from build123d import *

# Parameters (mm, degrees)
SKETCH1_W             = 15.24
SKETCH1_H             = 12.7
MAIN_BASE_DEPTH       = 2.54
ALIGNMENTPINS_START   = 1.778
SKETCH2_R             = 0.381
ALIGNMENTPINS_DEPTH   = 1.27
ALIGNMENTPINS_2_DEPTH = 1.27
SKETCH7_W             = 7.62
SKETCH7_H             = 12.7
PCBOARDEDGES_DEPTH    = 1.778
SKETCH12_W            = 4.379010271
SKETCH12_H            = 3.048
CONNECTORALIGN_DEPTH  = 2.54
SKETCH13_W            = 3.302
SKETCH13_H            = 5.08
LEDHOLE_DEPTH         = 5.318
SKETCH14_W            = 11.999010271
SKETCH14_H            = 6.858
SHOULDER_DEPTH        = 2.54
SKETCH15_W            = 11.999010271
SKETCH15_H            = 6.858
SHOULDER2_DEPTH       = 2.54
PCB_CLIP_START        = -4.37901
SKETCH17_R            = 0.254
PCB_CLIP_DEPTH        = 4.37901
SKETCH18_W            = 4.572
SKETCH18_H            = 2.54
NUNCHUCKCLIP_DEPTH    = 1.27
SKETCH19_W            = 4.572
SKETCH19_H            = 2.54
NUNCHUCKCLIP2_DEPTH   = 1.27
CUT_EXTRUDE1_DEPTH    = 0.508


with BuildPart() as part:
    # Sketch1 → Main Base (new body)
    with BuildSketch(Plane(origin=(0, 0, 0), x_dir=(1, 0, 0), z_dir=(0, 1, 0))):
        with Locations((7.62, 6.35)):
            Rectangle(SKETCH1_W, SKETCH1_H)
    extrude(amount=MAIN_BASE_DEPTH)



with BuildPart() as body_2:
    # Sketch2 → AlignmentPins (new body)
    with BuildSketch(Plane(origin=(0, 2.54, 0), x_dir=(-1, 0, 0), z_dir=(0, 1, 0)).offset(ALIGNMENTPINS_START)):
        with Locations((-0.762, -6.35)):
            Circle(SKETCH2_R)
    extrude(amount=ALIGNMENTPINS_DEPTH)


with BuildPart() as body_3:
    # Sketch2 → AlignmentPins 2 (new body)
    with BuildSketch(Plane(origin=(0, 2.54, 0), x_dir=(-1, 0, 0), z_dir=(0, 1, 0)).offset(ALIGNMENTPINS_START)):
        with Locations((-5.588, -6.35)):
            Circle(SKETCH2_R)
    extrude(amount=ALIGNMENTPINS_2_DEPTH)


with BuildPart() as part_1:
    add(part.part)

    add(body_2.part)  # PCBoardEdges merges body 2

    add(body_3.part)  # PCBoardEdges merges body 3
    # Sketch7 → PCBoardEdges (add)
    with BuildSketch(Plane(origin=(0, 2.54, 0), x_dir=(1, 0, 0), z_dir=(0, 1, 0))):
        with Locations((3.81, 6.35)):
            Rectangle(SKETCH7_W, SKETCH7_H)
    extrude(amount=PCBOARDEDGES_DEPTH)

    # Sketch12 → ConnectorAlign (add)
    with BuildSketch(Plane(origin=(0, 4.318, 0), x_dir=(1, 0, 0), z_dir=(0, 1, 0))):
        with Locations((5.430494864, 1.524)):
            Rectangle(SKETCH12_W, SKETCH12_H)
        with Locations((5.430494864, 11.176)):
            Rectangle(SKETCH12_W, SKETCH12_H)
    extrude(amount=CONNECTORALIGN_DEPTH)

    # Sketch13 → LEDHole (cut, through all)
    with BuildSketch(Plane(origin=(0, 4.318, 0), x_dir=(1, 0, 0), z_dir=(0, 1, 0))):
        with Locations((3.175, 6.35)):
            Rectangle(SKETCH13_W, SKETCH13_H)
    extrude(amount=-LEDHOLE_DEPTH, mode=Mode.SUBTRACT)

    # Sketch14 → Shoulder (add)
    with BuildSketch(Plane.XY):
        with Locations((9.240494865, 3.429)):
            Rectangle(SKETCH14_W, SKETCH14_H)
    extrude(amount=SHOULDER_DEPTH)

    # Sketch15 → Shoulder2 (add)
    with BuildSketch(Plane(origin=(0, 0, -12.7), x_dir=(-1, 0, 0), z_dir=(0, 0, -1))):
        with Locations((-9.240494865, 3.429)):
            Rectangle(SKETCH15_W, SKETCH15_H)
    extrude(amount=SHOULDER2_DEPTH)

    # Sketch17 → PCB_Clip (add)
    with BuildSketch(Plane(origin=(7.62, 0, 0), x_dir=(0, 0, -1), z_dir=(1, 0, 0)).offset(PCB_CLIP_START)):
        with Locations((3.048, 6.477)):
            Circle(SKETCH17_R)
        with Locations((9.652, 6.477)):
            Circle(SKETCH17_R)
    extrude(amount=PCB_CLIP_DEPTH)

    # Sketch18 → NunchuckClip (cut)
    with BuildSketch(Plane(origin=(0, 0, 0), x_dir=(-1, 0, 0), z_dir=(0, 0, -1))):
        with Locations((-9.906, 5.588)):
            Rectangle(SKETCH18_W, SKETCH18_H)
    extrude(amount=-NUNCHUCKCLIP_DEPTH, mode=Mode.SUBTRACT)

    # Sketch19 → NunchuckClip2 (cut)
    with BuildSketch(Plane.XY.offset(-12.7)):
        with Locations((9.906, 5.588)):
            Rectangle(SKETCH19_W, SKETCH19_H)
    extrude(amount=-NUNCHUCKCLIP2_DEPTH, mode=Mode.SUBTRACT)

    # Sketch20 → Cut-Extrude1 (cut)
    with BuildSketch(Plane.XZ):
        Polygon((8.217257779, -3.407193662), (8.217257779, -5.712243662), (6.016982779, -5.712243662), (6.016982779, -0.892593662), (14.398982779, -0.892593662), (14.398982779, -5.712243662), (12.198707779, -5.712243662), (12.198707779, -3.407193662), (11.255732779, -3.407193662), (11.255732779, -5.083593662), (9.055457779, -5.083593662), (9.055457779, -3.407193662), align=None)
        with BuildLine():
            Line((14.398982779, -7.493418662), (14.398982779, -11.893968662))
            Line((14.398982779, -11.893968662), (12.932132779, -11.893968662))
            Line((12.932132779, -11.893968662), (12.932132779, -9.819751084))
            Line((12.932132779, -9.819751084), (11.781244888, -9.62002374))
            add(Edge.make_bspline(
                [(11.781244888, -9.62002374), (11.770251243, -9.701615614), (11.748663963, -9.861830588), (11.690486481, -10.092391141), (11.615599165, -10.308891021), (11.520125231, -10.50985122), (11.405471862, -10.695560634), (11.270958242, -10.865311588), (11.120486873, -11.022229739), (10.949196623, -11.16103415), (10.761135353, -11.283987594), (10.557944594, -11.392930954), (10.337872373, -11.481879106), (10.102990479, -11.555971833), (9.853586477, -11.614857534), (9.588035638, -11.655012226), (9.307512918, -11.680069087), (9.114994844, -11.682943238), (9.016167154, -11.684418662)],
                knots=[0, 0, 0, 0, 0.000246818, 0.000484656, 0.000711955, 0.000933104, 0.001150717, 0.001365234, 0.001581735, 0.001801627, 0.002025024, 0.00225499, 0.002492123, 0.002735986, 0.002993304, 0.003260037, 0.003541058, 0.003837488, 0.003837488, 0.003837488, 0.003837488], degree=3))
            add(Edge.make_bspline(
                [(9.016167154, -11.684418662), (8.905845682, -11.682210565), (8.68961718, -11.677882727), (8.372872854, -11.644171577), (8.070289394, -11.591506566), (7.783499686, -11.513120981), (7.50963283, -11.418624818), (7.253853676, -11.294705499), (7.009895928, -11.155322531), (6.785472567, -10.99155228), (6.581476114, -10.81250602), (6.401376691, -10.621361865), (6.251345496, -10.416180814), (6.127577636, -10.200488598), (6.029896075, -9.973283881), (5.961530212, -9.734567465), (5.918899529, -9.48458455), (5.914467439, -9.314058562), (5.912207779, -9.22711749)],
                knots=[0, 0, 0, 0, 0.000330895, 0.000648549, 0.000954583, 0.00125123, 0.001539645, 0.00182231, 0.002102538, 0.002381539, 0.002654132, 0.002915916, 0.003167717, 0.003414839, 0.003660542, 0.00390768, 0.004158249, 0.004418878, 0.004418878, 0.004418878, 0.004418878], degree=3))
            add(Edge.make_bspline(
                [(5.912207779, -9.22711749), (5.91445515, -9.141879038), (5.918894654, -8.973497236), (5.952975516, -8.724244798), (6.006861153, -8.48157511), (6.081680985, -8.244815631), (6.181740166, -8.016042881), (6.300749021, -7.793180228), (6.443204901, -7.577175879), (6.60469356, -7.3712837), (6.778629295, -7.179505186), (6.962203599, -7.01236275), (7.15024709, -6.869703261), (7.343165184, -6.752025997), (7.544148349, -6.663616031), (7.748263448, -6.596817328), (7.959336029, -6.558322833), (8.101419593, -6.553084662), (8.173055826, -6.550443662)],
                knots=[0, 0, 0, 0, 0.000255646, 0.000505008, 0.000753251, 0.00100073, 0.001248584, 0.001501277, 0.001757823, 0.002023741, 0.002285618, 0.002533617, 0.002767397, 0.002992849, 0.00320977, 0.003424631, 0.003635926, 0.003850787, 0.003850787, 0.003850787, 0.003850787], degree=3))
            add(Edge.make_bspline(
                [(8.173055826, -6.550443662), (8.185703613, -6.55112084), (8.209065854, -6.552371684), (8.21468206, -6.574619572), (8.217257779, -6.584822959)],
                knots=[0, 0, 0, 0, 3.375e-05, 6.2341e-05, 6.2341e-05, 6.2341e-05, 6.2341e-05], degree=3))
            add(Edge.make_bspline(
                [(8.217257779, -6.584822959), (8.21379986, -6.598956726), (8.204910316, -6.635291506), (8.178023964, -6.661887625), (8.16159606, -6.678138193)],
                knots=[0, 0, 0, 0, 4.2972e-05, 0.000110472, 0.000110472, 0.000110472, 0.000110472], degree=3))
            add(Edge.make_bspline(
                [(8.16159606, -6.678138193), (8.136365772, -6.700405265), (8.077016572, -6.752784095), (7.993692338, -6.862131275), (7.902122779, -7.009388757), (7.800385555, -7.184339204), (7.708056874, -7.377085557), (7.639849213, -7.574659381), (7.596386201, -7.767637982), (7.591153517, -7.895938561), (7.588607779, -7.958357724)],
                knots=[0, 0, 0, 0, 0.000100772, 0.000237046, 0.000410069, 0.00062125, 0.000843879, 0.001049934, 0.0012474, 0.00143449, 0.00143449, 0.00143449, 0.00143449], degree=3))
            add(Edge.make_bspline(
                [(7.588607779, -7.958357724), (7.589364169, -8.003161205), (7.590845457, -8.090902724), (7.607861397, -8.218508769), (7.633961608, -8.339043342), (7.670022293, -8.453352628), (7.717335918, -8.560860294), (7.774738157, -8.661469601), (7.843243248, -8.754458019), (7.920801372, -8.840377114), (8.008056037, -8.917894183), (8.103416935, -8.984707761), (8.204925166, -9.042944891), (8.314460725, -9.087724989), (8.428623769, -9.127224479), (8.551689353, -9.149790175), (8.680576304, -9.167789672), (8.76943719, -9.169132909), (8.814802701, -9.169818662)],
                knots=[0, 0, 0, 0, 0.000134333, 0.000263072, 0.000385418, 0.000503982, 0.000622001, 0.000737136, 0.000850758, 0.00096782, 0.00108379, 0.001200071, 0.001316628, 0.001433998, 0.001554623, 0.001678233, 0.001808597, 0.001944566, 0.001944566, 0.001944566, 0.001944566], degree=3))
            add(Edge.make_bspline(
                [(8.814802701, -9.169818662), (8.855799497, -9.169091152), (8.935958333, -9.16766869), (9.052576868, -9.150249952), (9.16328584, -9.125037681), (9.265814181, -9.086505827), (9.363252497, -9.041250504), (9.451262049, -8.981147756), (9.533643551, -8.912152178), (9.609276284, -8.833428845), (9.67666913, -8.744332428), (9.73502713, -8.646476727), (9.785210532, -8.540365748), (9.823615634, -8.425214765), (9.85492271, -8.301566212), (9.87766612, -8.169699968), (9.890636219, -8.029012368), (9.892629227, -7.932736654), (9.893657779, -7.883050693)],
                knots=[0, 0, 0, 0, 0.000122881, 0.000240263, 0.000353034, 0.00046283, 0.000568268, 0.000674516, 0.000781419, 0.000890259, 0.001001257, 0.001115807, 0.001231522, 0.001352668, 0.00147933, 0.001613902, 0.001753672, 0.001902729, 0.001902729, 0.001902729, 0.001902729], degree=3))
            add(Edge.make_bspline(
                [(9.893657779, -7.883050693), (9.892472166, -7.825689716), (9.890150122, -7.713347192), (9.869778513, -7.548529099), (9.837864771, -7.391618982), (9.791184949, -7.242714697), (9.733050352, -7.101808236), (9.65950445, -6.969728078), (9.575093218, -6.844330987), (9.508174474, -6.768579517), (9.474557779, -6.730525693)],
                knots=[0, 0, 0, 0, 0.000172021, 0.000336907, 0.000497444, 0.000651749, 0.000804378, 0.000953849, 0.001104606, 0.001256786, 0.001256786, 0.001256786, 0.001256786], degree=3))
            Line((9.474557779, -6.730525693), (9.536767935, -6.655218662))
            Line((9.536767935, -6.655218662), (14.398982779, -7.493418662))
        make_face()
    extrude(amount=-CUT_EXTRUDE1_DEPTH, mode=Mode.SUBTRACT)


solid = part_1.part
Input: part model. Units: mm. Frame: model coordinates. A direction names the side the tool comes from. Coordinates: 2 decimals unless noted, no trailing zeros. Loops run counter-clockwise (first coordinate to the right, second up) from the corner with the lowest first, then second, coordinate; pieces in that order, holes last. Notation, with made-up numbers: (7.25, 35) -> (54.25, 35) arc R14 ccw to (54.25, 41) -> close; hole circle Ø10 at (-21.5, 68). An arc over 180 degrees is marked (long way). Write item = value, one per line. Start each with the question number.
Item 1: First-contact query: P1, Ø6, axis at x = 10, z = -9, coming from the +Y side; P2, Ø4, axis at y = 5, z = -4, coming from the +X side; P3, Ø1.4, axis at y = 5.5, z = -13, coming from the -X side; P4, Ø4, axis at x = 11.5, z = -3, coming from the +Y side. Flat tips, straight axial feed; report the tip coordinate or a pass-through.
Item 2: Reachability of faces 4 (the face through (3, 2, -3.81)), 5 (the face through (12, 4, 0)), 6 (the face through (10, 4.318, 1)), 7 (the face through (10, 0.508, -9)) from +Z, -Z, +X, -X, +Y, -Y: full face, straight path, thin tool, end or side. Return the list, or none.
Item 3: Cut plane C-C, the plane z = 0.75. Return loops of the section in (x, y), plus the area to 3 significant figures.
Item 4: Cut plane A-A, the plane z = -4.5. Return loops of the section in (x, y), plus the area to 3 significant figures.
Item 5: Mould query, pull axis X, two halves, no side actions, for faces 1 (the face through (15.24, 2, -6)), 2 (the face through (5, 5, -3.048)), 3 (the face through (4.826, 2, -6)). Classes: pulls with the +X half, pulls with the -X half, needs draft (parallel to the pull), parting line crosses it, or undercut.
Item 6: Cut plane D-D, the plane z = -6.35. Return loops of the section in (x, y).
Item 7: Cut plane B-B, the plane y = 2.75. Return loops of the section in (x, z).
Item 8: Material intervals for line 1 (Z direction, x = 13.75, y = 3.25); line 2 (X direction, y = 2.5, z = -6); line 3 (Z direction, x = 3, y = 3), sorted ascending.
Ans:
q1.P1 = 6.86
q1.P2 = 7.62
q1.P3 = 3.24
q1.P4 = 2.54
q2.face_4 = +Y, -Y
q2.face_5 = +X, +Y
q2.face_6 = +Y
q2.face_7 = -Y
q3.outline = (3.24, 0) -> (15.24, 0) -> (15.24, 6.86) -> (12.19, 6.86) -> (12.19, 4.32) -> (7.62, 4.32) -> (7.62, 6.86) -> (3.24, 6.86) -> close
q3.area = 70.7 mm²
q4.outline = (0, 0) -> (1.52, 0) -> (1.52, 4.32) -> (0, 4.32) -> close; (4.83, 0) -> (6.02, 0) -> (6.02, 0.51) -> (8.22, 0.51) -> (8.22, 0) -> (9.06, 0) -> (9.06, 0.51) -> (11.26, 0.51) -> (11.26, 0) -> (12.2, 0) -> (12.2, 0.51) -> (14.4, 0.51) -> (14.4, 0) -> (15.24, 0) -> (15.24, 2.54) -> (7.62, 2.54) -> (7.62, 4.32) -> (4.83, 4.32) -> close
q4.area = 34.6 mm²
q5.face_1 = pulls with the +X half
q5.face_2 = needs draft
q5.face_3 = undercut
q6.outline = (0, 0) -> (1.52, 0) -> (1.52, 4.32) -> (1.14, 4.32) -> (1.14, 5.59) -> (0.38, 5.59) -> (0.38, 4.32) -> (0, 4.32) -> close; (4.83, 0) -> (15.24, 0) -> (15.24, 2.54) -> (7.62, 2.54) -> (7.62, 4.32) -> (5.97, 4.32) -> (5.97, 5.59) -> (5.21, 5.59) -> (5.21, 4.32) -> (4.83, 4.32) -> close
q7.outline = (0, -12.7) -> (3.24, -12.7) -> (3.24, -15.24) -> (15.24, -15.24) -> (15.24, -12.7) -> (7.62, -12.7) -> (7.62, 0) -> (15.24, 0) -> (15.24, 2.54) -> (3.24, 2.54) -> (3.24, 0) -> (0, 0) -> close; hole (1.52, -8.89) -> (4.83, -8.89) -> (4.83, -3.81) -> (1.52, -3.81) -> close
q8.line_1 = -15.24 to -12.7, 0 to 2.54
q8.line_2 = 0 to 1.52, 4.83 to 15.24
q8.line_3 = -12.7 to -8.89, -3.81 to 0
